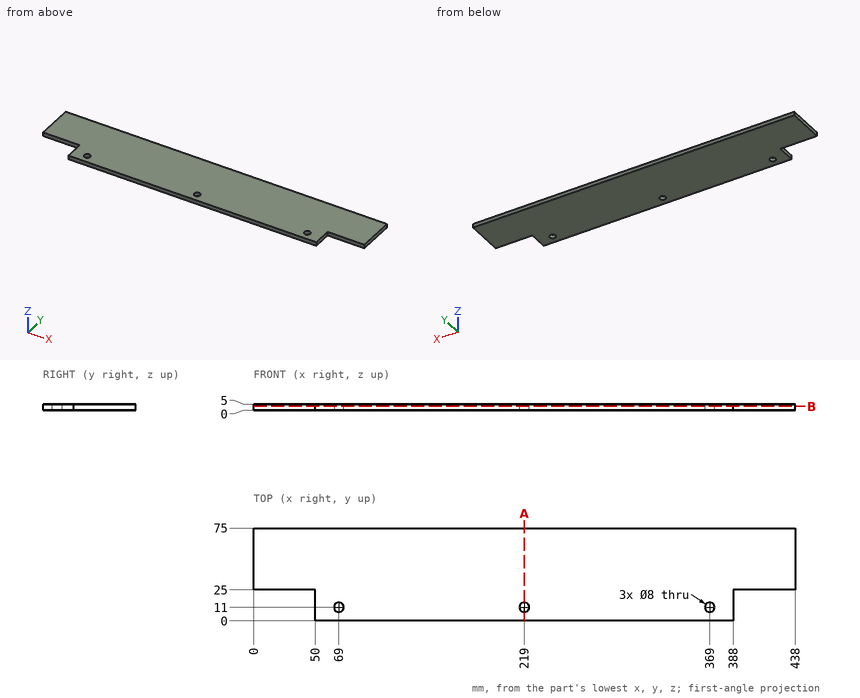
Part print with two shaded views. Sizes in mm from the minimum x, y, z corner. Coordinates: 2 decimals unless noted, no trailing zeros. Write each loop counter-clockwise with the first axis right and the second up, starting at its lowest first coordinate (ties: lowest second). Pieces come first, ordered by that corner, then holes. Notation, with made-up numbers: (-7.75, 3) - (40.25, 3) arc R18 ccw to (40.25, 11) - close; hole circle Ø1 at (62.5, -22). An arc over 180 degrees is marked (long way). One line per item, written item: value. Start each with the question number.
1. Slice it at A-A (x = 219). Write the cut outline in (y, z).
2. Slice it at B-B (z = 3.15). Write the cut outline in (x, y), plus the area to 3 significant figures.
3. Flat gauge pins, fed straight in: pin 1 (2.5 mm diameter, centred on y = 11, z = 3.5, fed in from +X); pin 2 (2.5 mm diameter, centred on x = 415, z = 3.5, fed in from -Y). Where does each tip first touch, or does it go through?
4. Probe line 1 (X direction, y = 14.5, z = 1.85); line 2 (Y direction, x = 219, z = 1.7); line 3 (X direction, y = 16, z = 3.05). List the from-to ranges inside material, lowest first. Write a range as from..to.
Answers below:
1. outline: (0, 0) - (7, 0) - (7, 5) - (0, 5) - close; (15, 0) - (75, 0) - (75, 5) - (15, 5) - close
2. outline: (0, 25) - (50, 25) - (50, 0) - (388, 0) - (388, 25) - (438, 25) - (438, 75) - (0, 75) - close; hole circle Ø8 at (69, 11); hole circle Ø8 at (219, 11); hole circle Ø8 at (369, 11)
2. area: 30,200 mm^2
3. pin 1: stops at x = 388
3. pin 2: stops at y = 25
4. line 1: x = 50..67.06, 70.94..217.06, 220.94..367.06, 370.94..388
4. line 2: y = 0..7, 15..75
4. line 3: x = 50..388
